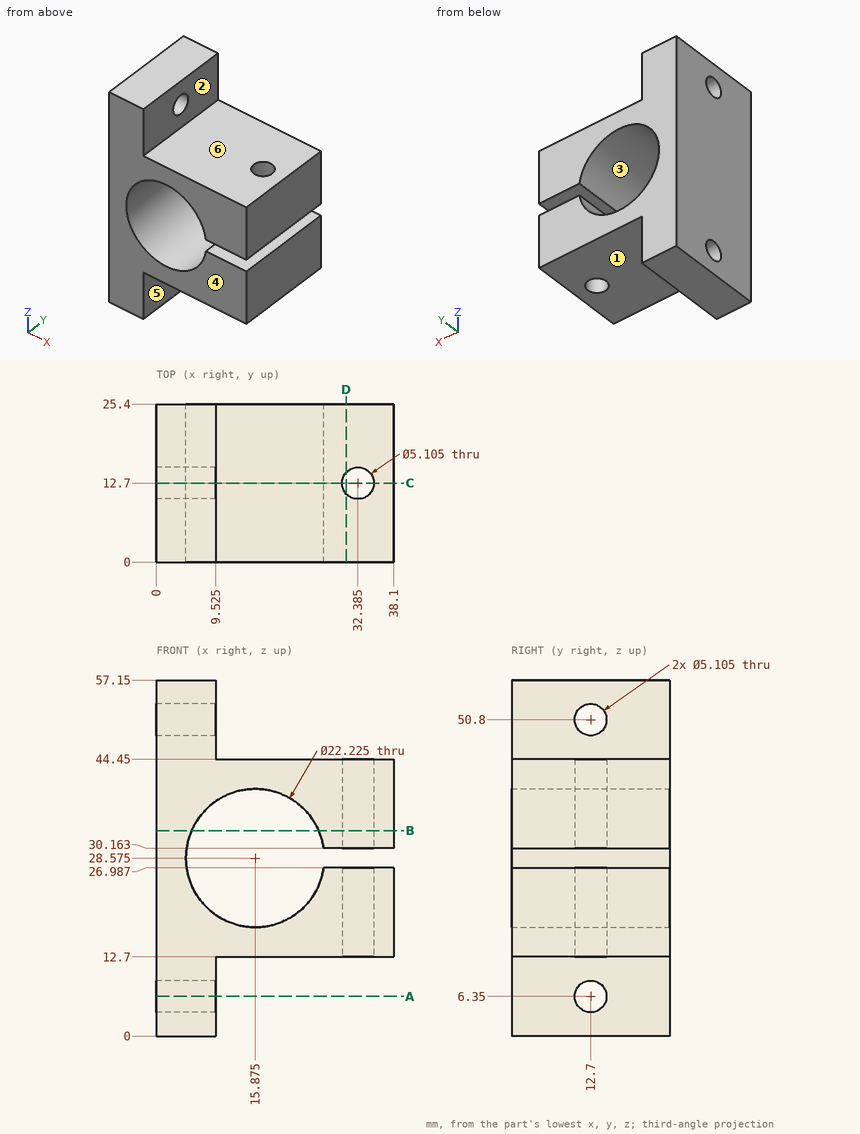
Job drawing, mm, ordinate dimensions from the low corner. One solid piece. A direction names the side the tool comes from. Round coordinates to 2 decimals unless told otherwise and drop trailing zeros. Write each loop counter-clockwise with the first axis right and the second up, starting at its lowest first coordinate (ties: lowest second). Pieces come first, ordered by that corner, then holes.
1) Mould opens along Z. For the marked faces 1, 2 and 3 say: +Z half, -Z half, draft (parallel to the pull), parting line (faces both ways), or undercut.
2) Band-saw the part on C-C, the plane y = 12.7. Give the number of separate pieces and of enclosed holes in the cut face, and give its area (3 significant figures).
3) Band-saw the part on B-B, the plane z = 33. List the corners of the cut face in (x, y) (1 decimal).
4) Pin check, flat tips, straight feed: pin 1 (12.5 mm diameter, centred on x = 18, y = 10, fed in from +Z); pin 2 (4 mm diameter, centred on y = 9, z = 48.5, fed in from +X) (1 decimal); pin 3 (12.5 mm diameter, centred on x = 32.5, y = 8, fed in from -Z). Stop position of each tip, or through.
5) Drill centre lines: probe 1 along Y at (x, z) = (5.75, 50.8); probe 2 along Z at (x, y) = (34, 20); probe 3 along X at (y, z) = (4.75, 51) (1 decimal). Where is each one in solid material? Low to high.
6) 3-axis set-ups, long thin cutter, end or side, ignore diameter. For the marked faces 4, 5 and 6: which of +Z, -Z, +X, -X, +Y, -Y reach the whole face in a straight line?
7) Band-saw the part on D-D, the plane x = 30.5. List the corners of the cut face in (y, z).
8) Band-saw the part on A-A, the plane z = 6.35. List the corners of the cut face in (x, y) (1 decimal), and give its area (3 significant figures).
Ans:
1. face 1: -Z half
1. face 2: draft
1. face 3: undercut
2. separate pieces: 5
2. enclosed holes: 0
2. area: 785 mm2
3. outline: (0, 0) - (5.7, 0) - (5.7, 25.4) - (0, 25.4) - close; (26.1, 0) - (38.1, 0) - (38.1, 25.4) - (26.1, 25.4) - close; hole circle Ø5.1 at (32.4, 12.7)
4. pin 1: stops at z = 44.45
4. pin 2: stops at x = 9.5
4. pin 3: stops at z = 12.7
5. probe 1: y = 0 to 10.15, 15.25 to 25.4
5. probe 2: z = 12.7 to 26.99, 30.16 to 44.45
5. probe 3: x = 0 to 9.5
6. face 4: +Z, -Z, +X, -X, -Y
6. face 5: -Z, +X, +Y, -Y
6. face 6: +Z, +X, +Y, -Y
7. outline: (0, 12.7) - (10.98, 12.7) - (10.98, 26.99) - (0, 26.99) - close; (0, 30.16) - (10.98, 30.16) - (10.98, 44.45) - (0, 44.45) - close; (14.42, 12.7) - (25.4, 12.7) - (25.4, 26.99) - (14.42, 26.99) - close; (14.42, 30.16) - (25.4, 30.16) - (25.4, 44.45) - (14.42, 44.45) - close
8. outline: (0, 0) - (9.5, 0) - (9.5, 10.1) - (0, 10.1) - close; (0, 15.3) - (9.5, 15.3) - (9.5, 25.4) - (0, 25.4) - close
8. area: 193 mm2
